```python
from build123d import *

# Parameters (mm, degrees)
F1_DEPTH = 82.5
F2_R     = 2.125
F2_W     = 45
F2_H     = 25.4
F3_DEPTH = 25.401
F4_R     = 3.25
F4_R_2   = 4.75
F4_R_3   = 2.125
F5_DEPTH = 5


with BuildPart() as f1:
    # F0 (on Right) → F1 (new body, symmetric)
    with BuildSketch(Plane.YZ):
        Polygon((-3.2, -25.4), (0, -25.4), (0, -3.2), (22.2, -3.2), (22.2, 0), (-3.2, 0), align=None)
    extrude(amount=F1_DEPTH, both=True)

    # F2 (on face) → F3 (cut, through all)
    with BuildSketch(Plane.XZ.offset(3.2)):
        with Locations((-67.5, -20.2)):
            Circle(F2_R)
        with Locations((-67.5, -7.7)):
            Circle(F2_R)
        with Locations((22.5, -7.7)):
            Circle(F2_R)
        with Locations((22.5, -20.2)):
            Circle(F2_R)
        with Locations((60, -12.7)):
            Rectangle(F2_W, F2_H)
    extrude(amount=-F3_DEPTH, mode=Mode.SUBTRACT)

    # F4 (on face) → F5 (cut)
    with BuildSketch(Plane.XY):
        with Locations((0, 11.1)):
            Circle(F4_R)
        with Locations((-45, 11.1)):
            Circle(F4_R_2)
        with Locations((-60, 11.1)):
            Circle(F4_R_3)
        with Locations((-30, 11.1)):
            Circle(F4_R_3)
        with Locations((-15, 11.1)):
            Circle(F4_R_3)
        with Locations((15, 11.1)):
            Circle(F4_R_3)
    extrude(amount=-F5_DEPTH, mode=Mode.SUBTRACT)


solid = f1.part
```
Read the model definition and answer for the solid it produces. Units are mm, in the model's axes. A direction names the side the tool comes from. Coordinates: 2 decimals unless noted, no trailing zeros. Write each loop counter-clockwise with the first axis right and the second up, starting at its lowest first coordinate (ties: lowest second). Pieces come first, ordered by that corner, then holes. Notation, with made-up numbers: (22, -27.5) -> (69, -27.5) arc R35 ccw to (69, 11.5) -> close; hole circle Ø6 at (39.25, 6.25). An arc over 180 degrees is marked (long way). Write item = value, one per line.
(1) Straight lines are drawn through the part: L1, parallel to Z at x = -67.5, y = -2.05 (3 decimals); L2, parallel to Y at x = -30, z = -2.45 (3 decimals); L3, parallel to Z at x = -39, y = 5.5. For each, find the intervals that lie inside material, in ascending order. Write a range as from..to.
From the geometry:
L1 = -25.4..-22.325, -18.075..-9.825, -5.575..0
L2 = -3.2..8.975, 13.225..22.2
L3 = -3.2..0
(2) For a pull along Y with two mould halves and no side action, classify faces 3 (the face through (-22, 0, -14)), 4 (the face through (-22, -3.2, -13)), 5 (the face through (13.31, 9.81, -1.58)) as +Y half, -Y half, draft (parallel to the pull), parting line (faces both ways), or undercut.
From the geometry:
face_3 = +Y half
face_4 = -Y half
face_5 = undercut
(3) Section B-B on z = -20.2 is taken. Write down the section's boundary in (x, y) (3 decimals).
From the geometry:
outline = (-82.5, -3.2) -> (-69.625, -3.2) -> (-69.625, 0) -> (-82.5, 0) -> close; (-65.375, -3.2) -> (20.375, -3.2) -> (20.375, 0) -> (-65.375, 0) -> close; (24.625, -3.2) -> (37.5, -3.2) -> (37.5, 0) -> (24.625, 0) -> close
(4) Given pin 1 Ø11 at (x, y) = (-51, 10) entering from -Z, flat-ended and moving along its own axis, determine where the tip first touches the part or whether it passes through.
From the geometry:
pin_1 = -3.2
(5) Section C-C on x = -60 is taken. Write down the section's boundary in (y, z) (3 decimals), plus the area to 3 significant figures.
From the geometry:
outline = (-3.2, -25.4) -> (0, -25.4) -> (0, -3.2) -> (8.975, -3.2) -> (8.975, 0) -> (-3.2, 0) -> close; (13.225, -3.2) -> (22.2, -3.2) -> (22.2, 0) -> (13.225, 0) -> close
area = 139 mm2
(6) Which of the six approach directions +Z, -Z, +X, -X, +Y, -Y give full straight-line access (tool end or side, diameter ignored) to faces 1 (the face through (-48.77, 8.21, -1.58)), 2 (the face through (-22, 11, -3.2))?
From the geometry:
face_1 = +Z, -Z
face_2 = -Z, +X, -X, +Y
(7) Section D-D on x = -21.5 is taken. Write down the section's boundary in (y, z).
From the geometry:
outline = (-3.2, -25.4) -> (0, -25.4) -> (0, -3.2) -> (22.2, -3.2) -> (22.2, 0) -> (-3.2, 0) -> close
(8) Section A-A on y = 11.1 is taken. Write down the section's boundary in (x, z) (3 decimals).
From the geometry:
outline = (-82.5, -3.2) -> (-62.125, -3.2) -> (-62.125, 0) -> (-82.5, 0) -> close; (-57.875, -3.2) -> (-49.75, -3.2) -> (-49.75, 0) -> (-57.875, 0) -> close; (-40.25, -3.2) -> (-32.125, -3.2) -> (-32.125, 0) -> (-40.25, 0) -> close; (-27.875, -3.2) -> (-17.125, -3.2) -> (-17.125, 0) -> (-27.875, 0) -> close; (-12.875, -3.2) -> (-3.25, -3.2) -> (-3.25, 0) -> (-12.875, 0) -> close; (3.25, -3.2) -> (12.875, -3.2) -> (12.875, 0) -> (3.25, 0) -> close; (17.125, -3.2) -> (37.5, -3.2) -> (37.5, 0) -> (17.125, 0) -> close
